Part model, mm, in its own coordinate system. Give positions to 0.01 mm unless a question says otherwise; leave off trailing zeros. Order: outer loops, then holes, each group sorted by start corner. A loop starts at its lowest first (then second) coordinate and runs counter-clockwise, first axis right, second up. Notation, with made-up numbers: (58, -14) - (89, -14) arc R23 ccw to (89, -6) - close; hole circle Ø9 at (21.25, -28.5). An arc over 180 degrees is marked (long way). Use one line per item in the form item = value. Start each with the question number.
1. Band-saw the part on C-C, the plane x = -7.75. List the corners of the cut face in (y, z).
2. Band-saw the part on B-B, the plane z = -295. List the corners of the cut face in (x, y), plus the area to 3 significant figures.
3. Band-saw the part on A-A, the plane y = 4.25. List the corners of the cut face in (x, z).
4. Drill centre lines: line 1 (Y direction, x = 4.75, z = -158); line 2 (X direction, y = -0.5, z = -266.5). Where is each one in solid material? Low to high.
5. Pin check, flat tips, straight feed: P1, Ø9, axis at x = -2, z = -164.5, coming from the +Y side; P2, Ø1, axis at y = -1, z = -73, coming from the +X side. Stop position of each tip, or through.
from build123d import *

# Parameters (mm, degrees)
BOSS_EXTRUDE1_DEPTH = 546


with BuildPart() as part:
    # Sketch1 → Boss-Extrude1 (new body)
    with BuildSketch(Plane.XY):
        Polygon((-12.500374185, 9.902439024), (-14.500374185, 9.902439024), (-14.500374185, -10.097560976), (5.499625815, -10.097560976), (5.499625815, -8.097560976), (-12.500374185, -8.097560976), align=None)
    extrude(amount=-BOSS_EXTRUDE1_DEPTH)


solid = part.part
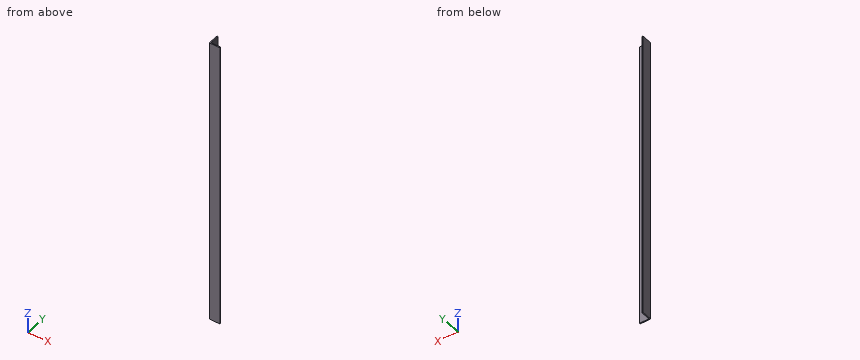
From the geometry:
q1.outline = (-10.1, -546) - (-8.1, -546) - (-8.1, 0) - (-10.1, 0) - close
q2.outline = (-14.5, -10.1) - (5.5, -10.1) - (5.5, -8.1) - (-12.5, -8.1) - (-12.5, 9.9) - (-14.5, 9.9) - close
q2.area = 76.0 mm²
q3.outline = (-14.5, -546) - (-12.5, -546) - (-12.5, 0) - (-14.5, 0) - close
q4.line_1 = -10.1 to -8.1
q4.line_2 = -14.5 to -12.5
q5.P1 = -8.1
q5.P2 = -12.5
